CAD build for the part. Positions are in the model's coordinates, mm. A direction names the side the tool comes from. Coordinates: 2 decimals unless noted, no trailing zeros. Order: outer loops, then holes, each group sorted by start corner. A loop starts at its lowest first (then second) coordinate and runs counter-clockwise, first axis right, second up. Notation, with made-up numbers: (38.5, 84.5) - (59.5, 84.5) arc R33 cw to (59.5, 112.5) - close; hole circle Ø8 at (2.5, 43.5). An arc over 180 degrees is marked (long way). Write each question's results on one line, items separated by ' | '. Start each with the question number.
Q1. Pin check, flat tips, straight feed: P1, Ø1.1, axis at x = 1, y = -44.5, coming from the -Z side; P2, Ø0.8, axis at x = 2, z = -2, coming from the -Y side; P3, Ø0.8, axis at x = -2.5, z = -2, coming from the -Y side; P4, Ø7.5, axis at x = -1, z = -11.5, coming from the +Y side. Stop position of each tip, or through.
Q2. Which spindle directions (+Z, -Z, +X, -X, +Y, -Y) get a long thin tool onto all of the face, cutting with end or side? Do faces 1 (the flat face through (0, -43, -4.268)), 2 (the cylindrical face through (1.615, 10.385, -13.105)), 3 (the flat face through (36.758, 23.263, -2.525)). Say none if no direction does.
Q3. Band-saw the part on A-A, the plane y = -34. Write the cut outline in (x, z).
Q4. Wall check: probe 1 along X at (y, z) = (5.5, -11); probe 2 along Y at (x, z) = (1, -11.5); probe 3 along Z at (x, y) = (0, -10.5). Give the ranges that are in metal, low to high.
```python
from build123d import *

# Parameters (mm, degrees)
F1_R          = 2.5
F2_DEPTH      = 30
F2_DEPTH_BACK = 2
F3_W          = 3.5355339059
F3_H          = 3.5355339059
F4_DEPTH      = 5
F5_COUNT      = 3
F6_R          = 1
F8_START      = 10
F7_R          = 3.5
F8_DEPTH      = 2
F9_START      = -10
F9_DEPTH      = 2


with BuildPart() as f11:
    # F10 (on Front) → F11 (revolve)
    with BuildSketch(Plane.XZ):
        Polygon((0, -5), (0, -10), (5, -5), (7, -5), (7, -15), (11, -15), (11, 0), (5, 0), align=None)
    revolve(axis=Axis((0, 0, -0.1335814595), (0, 0, -1)))

    # F1 (on offset) → F2 (join, two sides)
    with BuildSketch(Plane.XZ.offset(11)) as f2_sk:
        with Locations((0, -2.5)):
            Circle(F1_R)
    extrude(amount=F2_DEPTH)
    extrude(f2_sk.sketch, amount=-F2_DEPTH_BACK)

    # F3 (on face) → F4 (join)
    with BuildSketch(Plane.XZ.offset(41)):
        with Locations((0, -2.5)):
            Rectangle(F3_W, F3_H)
    extrude(amount=F4_DEPTH)

    # F5: F11 ×3 about axis
    f5_axis = Axis((0, 0, -15), (0, 0, 1))


with BuildPart() as f11_1:
    add(f11.part)
    for i in range(1, F5_COUNT):
        add(f11.part.rotate(f5_axis, i * 360 / F5_COUNT))

    # F6
    f6_edges = [f11_1.edges().sort_by_distance(p)[0] for p in [
        (-11, 0, -15),
        (-7, 0, -15),
    ]]
    fillet(f6_edges, radius=F6_R)

    # F7 (on Front) → F8 (cut)
    with BuildSketch(Plane.XZ.offset(F8_START)):
        with Locations((0, -10)):
            Circle(F7_R)
    extrude(amount=F8_DEPTH, mode=Mode.SUBTRACT)

    # F7 (on Front) → F9 (cut)
    with BuildSketch(Plane.XZ.offset(F9_START)):
        with Locations((0, -10)):
            Circle(F7_R)
    extrude(amount=-F9_DEPTH, mode=Mode.SUBTRACT)


solid = f11_1.part
```
Results below:
1) P1: stops at z = -4.27 | P2: stops at y = -46 | P3: stops at y = -41 | P4: stops at y = 11
2) face 1: -Z, +X, -X, -Y | face 2: +Y | face 3: +Z, -Z, +Y
3) outline: circle Ø5 at (0, -2.5)
4) probe 1: x = -9.53 to -4.33, 4.33 to 9.53 | probe 2: y = -10 to -6.93, 6.93 to 10 | probe 3: z = -14.87 to -13.5, -6.5 to 0
